Build history of the part. All positions in model axes, mm. Give positions to 0.01 mm unless a question says otherwise; leave off trailing zeros. Loops run counter-clockwise (first coordinate to the right, second up) from the corner with the lowest first, then second, coordinate; pieces in that order, holes last. Notation, with made-up numbers: M 29,42.5 L 74,42.5 A28 cw 74,69.5 Z; hole C -22,55.25 d9. An arc over 180 degrees is marked long. Put each result on its own line as item: value.
Autodesk Fusion 360 part; units mm, degrees
sketch "Sketch1" plane through (0, 0, 0) normal (0, 0, 1) x (1, 0, 0)
  circle A0 centre (0, 0) radius 5
  circle A1 centre (0, 0) radius 12.5
  dimension "d1" = 10
  dimension "d2" = 25
extrude "Extrude1" add sketch "Sketch1" along normal blind 1.5 makes body 1
copy_body "Body->Comp1" bodies 1 removing the originals makes body 2 in component "M10x25x1.5 washer"
component "M10x25x1.5 washer" placed x (1, 0, 0) y (0, 1, 0) z (0, 0, 1) at (0, 0, 0)
Q1. Slice it at A-A (x = 0). List the corners of the cut face in (y, z), and give its area (3 significant figures).
Here are the results:
outline: M -12.5,0 L -5,0 L -5,1.5 L -12.5,1.5 Z; M 5,0 L 12.5,0 L 12.5,1.5 L 5,1.5 Z
area: 22.5 mm²
Q2. Probe line 1 (Y direction, x = 0, z = 0.45); line 2 (X direction, y = 3.75, z = 1); line 3 (X direction, y = -3, z = 0.4). List the from-to ranges inside material, lowest first. Write a range as from..to.
Here are the results:
line 1: -12.5..-5, 5..12.5
line 2: -11.92..-3.31, 3.31..11.92
line 3: -12.13..-4, 4..12.13
Q3. Slice it at C-C (z = 1). List the corners of the cut face in (x, y).
Here are the results:
outline: C 0,0 d25; hole C 0,0 d10
Q4. Mould opens along Y. For faces 1 (the flat face through (-0.2, -5.4, 0)), 2 (the cylindrical face through (-1.08, 4.88, 0.74)), 3 (the cylindrical face through (11.923, -3.755, 0.74)) say: pulls with the +Y half, pulls with the -Y half, needs draft (parallel to the pull), parting line crosses it, or undercut.
Here are the results:
face 1: needs draft
face 2: undercut
face 3: parting line crosses it
Q5. Slice it at B-B (y = -1.5). List the corners of the cut face in (x, z).
Here are the results:
outline: M -12.41,0 L -4.77,0 L -4.77,1.5 L -12.41,1.5 Z; M 4.77,0 L 12.41,0 L 12.41,1.5 L 4.77,1.5 Z
Q6. Slice it at D-D (y = -9). List the corners of the cut face in (x, z).
Here are the results:
outline: M -8.67,0 L 8.67,0 L 8.67,1.5 L -8.67,1.5 Z
